For this review, take the finished solid that the model builds, in its own axes (mm). Face numbers are marked on the shaded views. Round coordinates to 2 decimals unless told otherwise and drop trailing zeros.
```python
from build123d import *

# Parameters (mm, degrees)
ESQUISSE1_W             = 324
ESQUISSE1_H             = 388
BOSS_EXTRU_1_DEPTH      = 8
ENL_V_MAT_EXTRU_1_DEPTH = 1
ESQUISSE3_R             = 2.25
ENL_V_MAT_EXTRU_2_DEPTH = 253.841847802
ENL_V_MAT_EXTRU_3_DEPTH = 1
ESQUISSE5_R             = 3.25
ENL_V_MAT_EXTRU_4_DEPTH = 253.841847802


with BuildPart() as part:
    # Esquisse1 → Boss.-Extru.1 (new body)
    with BuildSketch(Plane.XY):
        Rectangle(ESQUISSE1_W, ESQUISSE1_H)
    extrude(amount=BOSS_EXTRU_1_DEPTH)

    # Esquisse2 → Enlèv. mat.-Extru.1 (cut)
    with BuildSketch(Plane.XY.offset(8)):
        with BuildLine():
            Line((148, -114), (156.9, -114))
            ThreePointArc((156.9, -114), (160.48492424, -112.51507576), (159, -116.1))
            Line((159, -116.1), (159, -189))
            Line((159, -189), (148, -189))
            Line((148, -189), (148, -114))
        make_face()
    enl_v_mat_extru_1 = extrude(amount=-ENL_V_MAT_EXTRU_1_DEPTH, mode=Mode.SUBTRACT)

    # Symétrie1: Enlèv. mat.-Extru.1 across plane
    add(enl_v_mat_extru_1.mirror(Plane(origin=(0, 0, 0), x_dir=(0, 0, 1), z_dir=(1, 0, 0))), mode=Mode.SUBTRACT)

    # Esquisse3 → Enlèv. mat.-Extru.2 (cut, through all)
    with BuildSketch(Plane.XY.offset(7)):
        with Locations((154, -121)):
            Circle(ESQUISSE3_R)
        with Locations(Location((154, -181, 0), (0, 0, 180))):
            Circle(ESQUISSE3_R)
    enl_v_mat_extru_2 = extrude(amount=-ENL_V_MAT_EXTRU_2_DEPTH, mode=Mode.SUBTRACT)

    # Symétrie2: Enlèv. mat.-Extru.2 across plane
    add(enl_v_mat_extru_2.mirror(Plane(origin=(0, 0, 0), x_dir=(0, 0, 1), z_dir=(1, 0, 0))), mode=Mode.SUBTRACT)

    # Esquisse4 → Enlèv. mat.-Extru.3 (cut)
    with BuildSketch(Plane.XY.offset(8)):
        with BuildLine():
            Line((-34, 189), (31.9, 189))
            ThreePointArc((31.9, 189), (35.48492424, 190.48492424), (34, 186.9))
            Line((34, 186.9), (34, 172))
            Line((34, 172), (-34, 172))
            Line((-34, 172), (-34, 189))
        make_face()
        with BuildLine():
            Line((34, 143.1), (34, 158))
            Line((34, 158), (-34, 158))
            Line((-34, 158), (-34, 141))
            Line((-34, 141), (31.9, 141))
            ThreePointArc((31.9, 141), (35.48492424, 139.51507576), (34, 143.1))
        make_face()
    extrude(amount=-ENL_V_MAT_EXTRU_3_DEPTH, mode=Mode.SUBTRACT)

    # Esquisse5 → Enlèv. mat.-Extru.4 (cut, through all)
    with BuildSketch(Plane.XY.offset(7)):
        with Locations((-26.5, 181)):
            Circle(ESQUISSE5_R)
        with Locations(Location((26.5, 181, 0), (0, 0, 180))):
            Circle(ESQUISSE5_R)
        with Locations((26.5, 149)):
            Circle(ESQUISSE5_R)
        with Locations(Location((-26.5, 149, 0), (0, 0, 180))):
            Circle(ESQUISSE5_R)
    extrude(amount=-ENL_V_MAT_EXTRU_4_DEPTH, mode=Mode.SUBTRACT)


solid = part.part
```
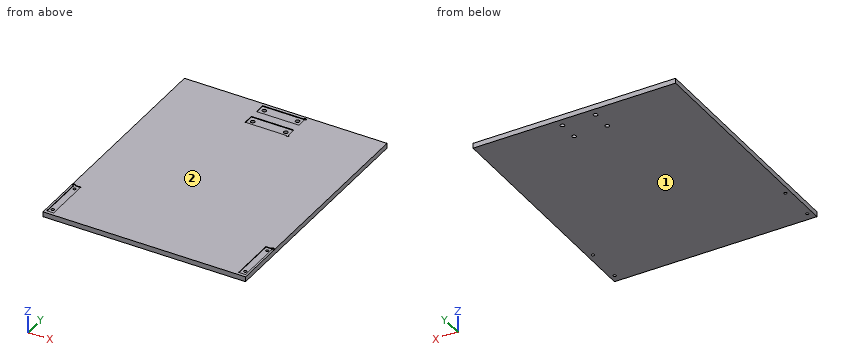
Q1. Wall thickness on line 1 (X direction, y = 181, z = 5.75); line 2 (Y direction, x = 9, z = 7.5); line 3 (X direction, y = -181, z = 2.75): over which ranges is each line inside the solid? List them lowest first.
Q2. Mouldability with a two-part tool opening along Z and no side actions: class the marked faces 1 and 2 as +Z half, -Z half, draft (parallel to the pull), parting line (faces both ways), or undercut.
Q3. Clearance check with flat-ended pins moving along their axes: pin 1 (3 mm diameter, centred on x = 24, y = 150.5, fed in from +Z); pin 2 (5 mm diameter, centred on x = 154, y = -121, fed in from -Z). State where each tip first meets the part, or that it passes through.
Working result:
1. line 1: x = -162 to -29.75, -23.25 to 23.25, 29.75 to 162
1. line 2: y = -194 to 141, 158 to 172, 189 to 194
1. line 3: x = -162 to -156.25, -151.75 to 151.75, 156.25 to 162
2. face 1: -Z half
2. face 2: +Z half
3. pin 1: stops at z = 7
3. pin 2: stops at z = 0
